```python
from build123d import *

# Parameters (mm, degrees)
SKETCH_1_W          = 210
SKETCH_1_H          = 120
SKETCH_1_R          = 3.25
SKETCH_1_R_2        = 30
EXTRUDE_1_DEPTH     = 6
SKETCH_2_R          = 2.5
CUT_EXTRUDE_1_DEPTH = 10
SKETCH_3_R          = 2
CUT_EXTRUDE_2_DEPTH = 20


with BuildPart() as part:
    # 草图1 → 凸台-拉伸1 (new body)
    with BuildSketch(Plane.XY):
        with Locations((-45, 0)):
            Rectangle(SKETCH_1_W, SKETCH_1_H)
        with Locations((26.516504294, 26.516504294)):
            Circle(SKETCH_1_R, mode=Mode.SUBTRACT)
        with Locations((26.516504294, -26.516504294)):
            Circle(SKETCH_1_R, mode=Mode.SUBTRACT)
        with Locations((-26.516504294, -26.516504294)):
            Circle(SKETCH_1_R, mode=Mode.SUBTRACT)
        with Locations((-26.516504294, 26.516504294)):
            Circle(SKETCH_1_R, mode=Mode.SUBTRACT)
        Circle(SKETCH_1_R_2, mode=Mode.SUBTRACT)
    extrude(amount=EXTRUDE_1_DEPTH)

    # 草图2 → 切除-拉伸1 (cut)
    with BuildSketch(Plane.XY.offset(6)):
        with Locations((-137, 40)):
            Circle(SKETCH_2_R)
        with Locations((-107, 40)):
            Circle(SKETCH_2_R)
        with Locations((-107, -40)):
            Circle(SKETCH_2_R)
        with Locations((-137, -40)):
            Circle(SKETCH_2_R)
    extrude(amount=-CUT_EXTRUDE_1_DEPTH, mode=Mode.SUBTRACT)

    # 草图3 → 切除-拉伸2 (cut)
    with BuildSketch(Plane(origin=(0, -60, 0), x_dir=(-1, 0, 0), z_dir=(0, -1, 0))):
        with Locations((-57, -3)):
            Circle(SKETCH_3_R)
        with Locations((11, -3)):
            Circle(SKETCH_3_R)
        with Locations((79, -3)):
            Circle(SKETCH_3_R)
        with Locations((147, -3)):
            Circle(SKETCH_3_R)
    cut_extrude_2 = extrude(amount=-CUT_EXTRUDE_2_DEPTH, mode=Mode.SUBTRACT)

    # 镜向3: 切除-拉伸2 across plane
    add(cut_extrude_2.mirror(Plane(origin=(0, 0, 0), x_dir=(0, 0, 1), z_dir=(0, -1, 0))), mode=Mode.SUBTRACT)


solid = part.part
```
Could you check a few things on this model? Use its own coordinates, in mm. A direction names the side the tool comes from. Coordinates: 2 decimals unless noted, no trailing zeros. Loops run counter-clockwise (first coordinate to the right, second up) from the corner with the lowest first, then second, coordinate; pieces in that order, holes last.
1) Please list where these lines run through material, in increasing order: line 1 along Y through (x, z) = (-137, 3.7); line 2 along X through (y, z) = (53.25, 3); line 3 along Z through (x, y) = (-79, -50.25).
Reported:
line 1: y = -60 to -42.5, -37.5 to 37.5, 42.5 to 60
line 2: x = -150 to -149, -145 to -81, -77 to -13, -9 to 55, 59 to 60
line 3: z = 0 to 1, 5 to 6
2) Imagine slicing it at C-C (x = -107). List the corners of the cut face in (y, z) for me.
Reported:
outline: (-60, 0) - (-42.5, 0) - (-42.5, 6) - (-60, 6) - close; (-37.5, 0) - (37.5, 0) - (37.5, 6) - (-37.5, 6) - close; (42.5, 0) - (60, 0) - (60, 6) - (42.5, 6) - close
3) Which directions (+Z, -Z, +X, -X, +Y, -Y) give clear straight access to the entire face, cutting with the end or side of a thin tool? Please do faces 4 (the face through (-9.4, 50.1, 4.2)), 5 (the face through (55.153, -50.14, 3.766)), 6 (the face through (23.27, 26.66, 2.96)).
Reported:
face 4: +Y
face 5: -Y
face 6: +Z, -Z
4) Thinking about a two-plate mould opening in Y: for faces 1 (the face through (-134.69, 39.04, 3.04)), 2 (the face through (-79, 40, 3)), 3 (the face through (55.153, 50.14, 3.766)), which applies, released by +Y, released by -Y, zero draft, split by the parting line, or undercut?
Reported:
face 1: undercut
face 2: released by +Y
face 3: zero draft
5) Imagine slicing it at D-D (x = 57). List the corners of the cut face in (y, z) for me.
Reported:
outline: (-60, 0) - (60, 0) - (60, 1) - (40, 1) - (40, 5) - (60, 5) - (60, 6) - (-60, 6) - (-60, 5) - (-40, 5) - (-40, 1) - (-60, 1) - close
6) Imagine slicing it at B-B (y = -5). List the corners of the cut face in (x, z) for me, and give its area (3 significant figures).
Reported:
outline: (-150, 0) - (-29.58, 0) - (-29.58, 6) - (-150, 6) - close; (29.58, 0) - (60, 0) - (60, 6) - (29.58, 6) - close
area: 905 mm2
7) Imagine slicing it at A-A (x = 0). List the corners of the cut face in (y, z) for me, and give its area (3 significant figures).
Reported:
outline: (-60, 0) - (-30, 0) - (-30, 6) - (-60, 6) - close; (30, 0) - (60, 0) - (60, 6) - (30, 6) - close
area: 360 mm2
8) Will these pins go through, and if not, where does the flat tip stop? pin 1 Ø4.5 at (x, y) = (-107, 40) entering from -Z; pin 2 Ø1.2 at (x, z) = (-147.5, 3.5) entering from +Y; pin 3 Ø1.2 at (x, z) = (-146, 3.5) entering from -Y.
Reported:
pin 1: passes through
pin 2: stops at y = 40
pin 3: stops at y = -40
